Check sheet for the drawn part. Datum: minimum x, y, z corner. Units: mm. Round coordinates to 2 decimals unless told otherwise and drop trailing zeros. Write each loop counter-clockwise with the first axis right and the second up, starting at its lowest first coordinate (ties: lowest second). Pieces come first, ordered by that corner, then holes. Notation, with made-up numbers: (32, -29.5) -> (38, -29.5) arc R13 cw to (38, -13.5) -> close; hole circle Ø1 at (47.5, 29.5). An arc over 180 degrees is marked (long way). Use a Markdown table: item, result.
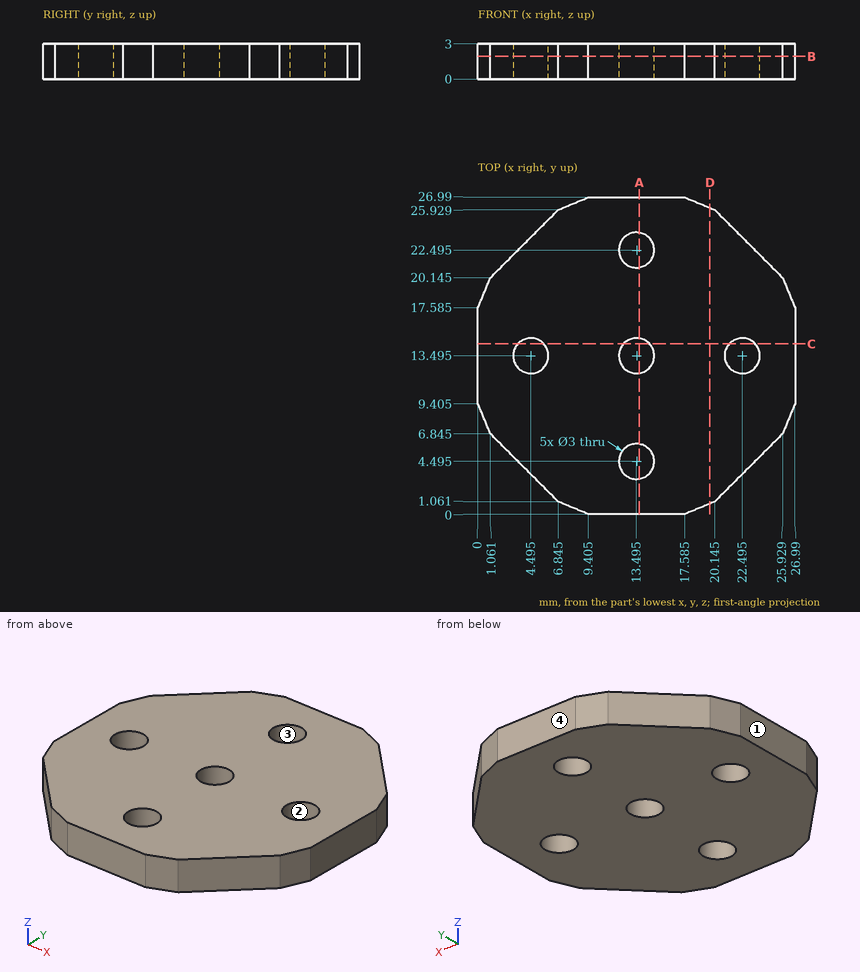
(1) Thickness scan on line 1 (X direction, y = 13.5, z = 0.7) (1 decimal); line 2 (Y direction, x = 14.5, z = 1.85). Record the ranges inside material, lowest first.
A:
| item | result |
|---|---|
| line 1 | x = 0 to 3, 6 to 12, 15 to 21, 24 to 27 |
| line 2 | y = 0 to 3.38, 5.61 to 12.38, 14.61 to 21.38, 23.61 to 26.99 |
(2) Section check D-D on x = 19.75. Record the cut outline in (y, z).
A:
| item | result |
|---|---|
| outline | (0.9, 0) -> (26.09, 0) -> (26.09, 3) -> (0.9, 3) -> close |
(3) Release check for a two-part mould opening along Y. For the marked faces 1, 2, 3 and 4 record: +Y half, -Y half, draft (parallel to the pull), parting line (faces both ways), or undercut.
A:
| item | result |
|---|---|
| face 1 | draft |
| face 2 | undercut |
| face 3 | undercut |
| face 4 | +Y half |
(4) Section check C-C on y = 14.5. Record the cut outline in (x, z).
A:
| item | result |
|---|---|
| outline | (0, 0) -> (3.38, 0) -> (3.38, 3) -> (0, 3) -> close; (5.61, 0) -> (12.38, 0) -> (12.38, 3) -> (5.61, 3) -> close; (14.61, 0) -> (21.38, 0) -> (21.38, 3) -> (14.61, 3) -> close; (23.61, 0) -> (26.99, 0) -> (26.99, 3) -> (23.61, 3) -> close |
(5) Section check B-B on z = 1.95. Record the cut outline in (x, y) (1 decimal).
A:
| item | result |
|---|---|
| outline | (0, 9.4) -> (1.1, 6.8) -> (6.8, 1.1) -> (9.4, 0) -> (17.6, 0) -> (20.1, 1.1) -> (25.9, 6.8) -> (27, 9.4) -> (27, 17.6) -> (25.9, 20.1) -> (20.1, 25.9) -> (17.6, 27) -> (9.4, 27) -> (6.8, 25.9) -> (1.1, 20.1) -> (0, 17.6) -> close; hole circle Ø3 at (4.5, 13.5); hole circle Ø3 at (13.5, 4.5); hole circle Ø3 at (13.5, 13.5); hole circle Ø3 at (13.5, 22.5); hole circle Ø3 at (22.5, 13.5) |
(6) Gauge pin test, flat end, axial feed: pin 1 Ø4 at (x, y) = (13.495, 13.495) entering from -Z. Record the tip position at first contact, or that the pin passes through.
A:
| item | result |
|---|---|
| pin 1 | stops at z = 0 |
(7) Section check A-A on x = 13.75. Record the cut outline in (y, z).
A:
| item | result |
|---|---|
| outline | (0, 0) -> (3.02, 0) -> (3.02, 3) -> (0, 3) -> close; (5.97, 0) -> (12.02, 0) -> (12.02, 3) -> (5.97, 3) -> close; (14.97, 0) -> (21.02, 0) -> (21.02, 3) -> (14.97, 3) -> close; (23.97, 0) -> (26.99, 0) -> (26.99, 3) -> (23.97, 3) -> close |
